Part model, mm, in its own coordinate system. Face numbers are marked on the shaded views. A direction names the side the tool comes from. Give positions to 0.01 mm unless a question says otherwise; leave off trailing zeros. Write each loop counter-clockwise with the first axis right and the second up, starting at its lowest first coordinate (ties: lowest second). Pieces come first, ordered by that corner, then holes. Notation, with made-up numbers: M -3,14.25 L 26,14.25 A10 cw 26,28.25 Z; hole C 80.25,19 d8. An arc over 180 degrees is marked long. Answer as CSV lines item,"result". Start each with the question number.
Item 1: Band-saw the part on C-C, the plane y = 21.5. List the corners of the cut face in (x, z).
Item 2: Band-saw the part on B-B, the plane x = -43. List the corners of the cut face in (y, z), then the cut area to 3 significant figures.
Item 3: Wall check: L1, parallel to Z at x = -42, y = 4.5; L2, parallel to Z at x = -44.5, y = 36; L3, parallel to Y at x = -37.5, z = 3.5. Give the ranges that are in metal, low to high. Write a range as from..to.
Item 4: Band-saw the part on D-D, the plane z = 2.75. List the corners of the cut face in (x, y), then the cut area to 3 significant figures.
Item 5: Band-saw the part on A-A, the plane z = -12.75. List the corners of the cut face in (x, y), then the cut area to 3 significant figures.
Item 6: Two-plate mould, pull along X, no slides. Class the marked faces 1, 2 and 3: +X half, -X half, draft (parallel to the pull), parting line (faces both ways), or undercut.
Item 7: 3-axis set-ups, long thin cutter, end or side, ignore diameter. For the marked faces 4, 5 and 6: which of +Z, -Z, +X, -X, +Y, -Y reach the whole face in a straight line?
Item 8: Pin check, flat tips, straight feed: pin 1 (1.5 mm diameter, centred on x = -40, y = 27, fed in from -Z); pin 2 (3 mm diameter, centred on x = -44.5, z = -12.5, fed in from +Y); pin 3 (1 mm diameter, centred on x = -41.5, y = 36, fed in from +Z). Stop position of each tip, or through.
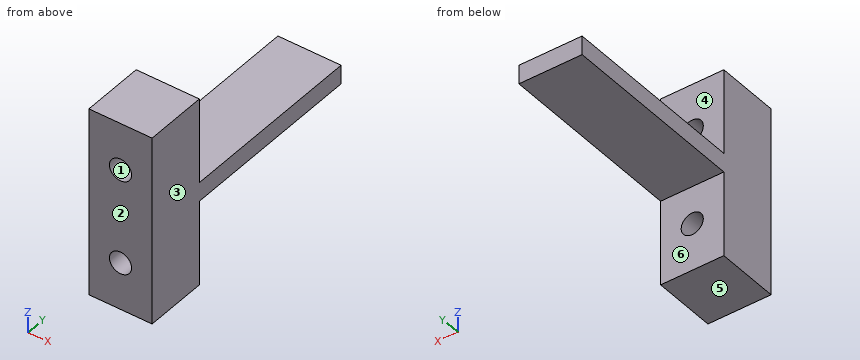
from build123d import *

# Parameters (mm, degrees)
SKETCH2_W           = 10
SKETCH2_H           = 30
SKETCH2_R           = 1.75
BOSS_EXTRUDE1_DEPTH = 10
SKETCH4_W           = 10
SKETCH4_H           = 1.5
BOSS_EXTRUDE3_DEPTH = 30


with BuildPart() as part:
    # Sketch2 → Boss-Extrude1 (new body)
    with BuildSketch(Plane(origin=(0, 0, 0), x_dir=(1, 0, 0), z_dir=(0, 1, 0))):
        with Locations((-41.876032971, 5.874496677)):
            Rectangle(SKETCH2_W, SKETCH2_H)
        with Locations(Location((-41.876032971, -1.625503323, 0), (0, 0, 270))):
            Circle(SKETCH2_R, mode=Mode.SUBTRACT)
        with Locations(Location((-41.876032971, 13.374496677, 0), (0, 0, 270))):
            Circle(SKETCH2_R, mode=Mode.SUBTRACT)
    extrude(amount=BOSS_EXTRUDE1_DEPTH)

    # Sketch4 → Boss-Extrude3 (add)
    with BuildSketch(Plane(origin=(0, 10, 0), x_dir=(1, 0, 0), z_dir=(0, 1, 0))):
        with Locations((-41.876032971, 6.624496677)):
            Rectangle(SKETCH4_W, SKETCH4_H)
        with Locations((-41.876032971, 5.124496677)):
            Rectangle(SKETCH4_W, SKETCH4_H)
    extrude(amount=BOSS_EXTRUDE3_DEPTH)


solid = part.part
Output:
1,outline,"M -46.88,-7.37 L -36.88,-7.37 L -36.88,-4.37 L -46.88,-4.37 Z"
2,outline,"M 0,-20.87 L 10,-20.87 L 10,-14.72 L 0,-14.72 Z; M 0,-12.03 L 10,-12.03 L 10,-7.37 L 40,-7.37 L 40,-4.37 L 10,-4.37 L 10,0.28 L 0,0.28 Z; M 0,2.97 L 10,2.97 L 10,9.13 L 0,9.13 Z"
2,area,"336 mm²"
3,L1,"-20.87..-15.12, -11.63..-0.12, 3.37..9.13"
3,L2,"-7.37..-4.37"
3,L3,"0..10"
4,outline,"M -46.88,0 L -43.22,0 L -43.22,10 L -46.88,10 Z; M -40.54,0 L -36.88,0 L -36.88,10 L -40.54,10 Z"
4,area,"73.2 mm²"
5,outline,"M -46.88,0 L -43.51,0 L -43.51,10 L -46.88,10 Z; M -40.24,0 L -36.88,0 L -36.88,10 L -40.24,10 Z"
5,area,"67.3 mm²"
6,face 1,"undercut"
6,face 2,"draft"
6,face 3,"+X half"
7,face 4,"+Z, +X, -X, +Y"
7,face 5,"-Z, +X, -X, +Y, -Y"
7,face 6,"-Z, +X, -X, +Y"
8,pin 1,"z = -7.37"
8,pin 2,"y = 10"
8,pin 3,"z = -4.37"
